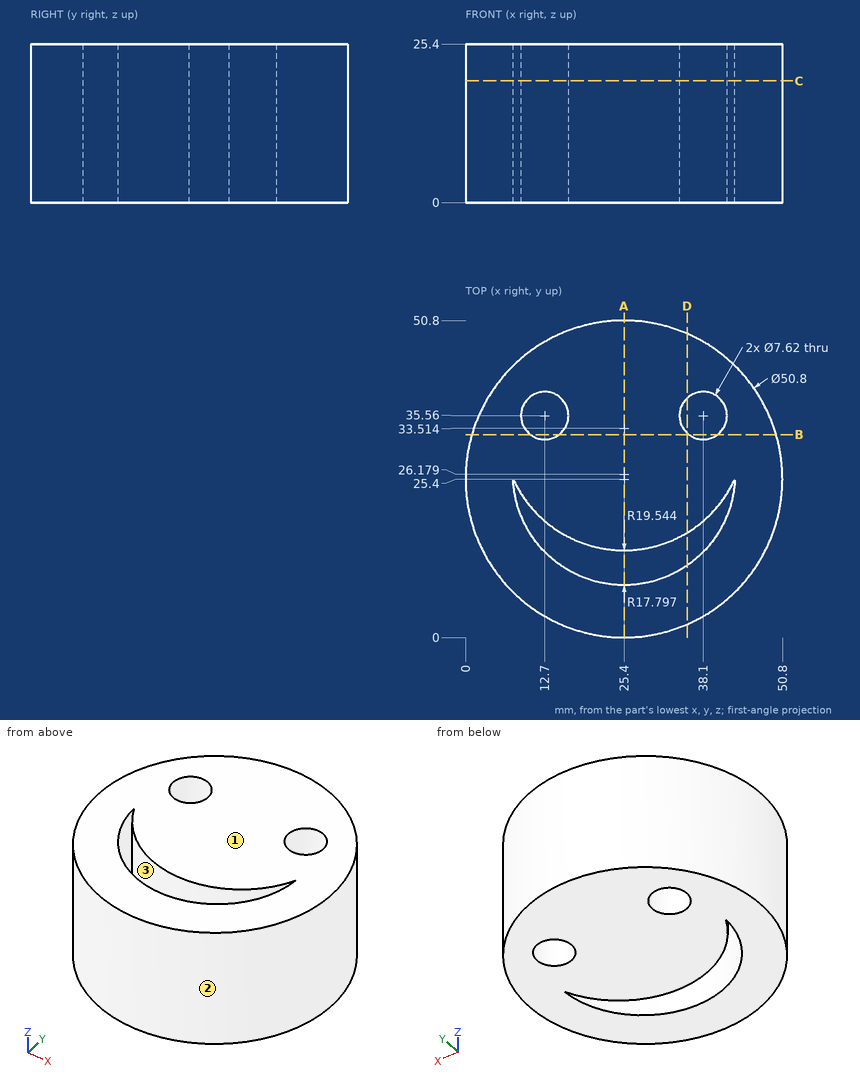
For this review, use the dimensioned drawing (mm, ordinates from the lowest corner) and the shaded views. Give positions to 0.01 mm unless a question says otherwise; leave off trailing zeros. Order: outer loops, then holes, each group sorted by start corner. A loop starts at its lowest first (then second) coordinate and runs counter-clockwise, first axis right, second up.
1) Take a section at B-B (y = 32.5). Give the boundary of the cut face in (x, z), then the cut area to 3 significant figures.
2) The part is to be moulded in two halves that separate along X. For the marked faces 1, 2 and 3, say which applies: released by +X, released by -X, zero draft, split by the parting line, or undercut.
3) Wall thickness on line 1 (Y direction, x = 12, z = 9.5) (1 decimal); line 2 (Y direction, x = 12.7, z = 13.5); line 3 (X direction, y = 16.5, z = 15.75) (1 decimal): over which ranges is each line inside the solid? List them lowest first.
4) Take a section at A-A (x = 25.4). Give the boundary of the cut face in (y, z), then the cut area to 3 significant figures.
5) Take a section at D-D (x = 35.5). Give the boundary of the cut face in (y, z) (1 decimal), then the cut area to 3 significant figures.
6) Insertion check: pin 1 (4 mm diameter, centred on y = 41, z = 19, fed in from -X); pin 2 (12 mm diameter, centred on x = 17, z = 21.5, fed in from -Y); pin 3 (6 mm diameter, centred on y = 40.5, z = 11, fed in from -X). Each pin has a flat end and moves straight along its axis. Give the tip position at first contact, or say it passes through.
7) Take a section at C-C (z = 19.5). Give the boundary of the cut face in (x, y).
Derived:
1. outline: (1.01, 0) - (10.43, 0) - (10.43, 25.4) - (1.01, 25.4) - close; (14.97, 0) - (35.83, 0) - (35.83, 25.4) - (14.97, 25.4) - close; (40.37, 0) - (49.79, 0) - (49.79, 25.4) - (40.37, 25.4) - close
1. area: 1,010 mm2
2. face 1: zero draft
2. face 2: split by the parting line
2. face 3: undercut
3. line 1: y = 3.8 to 14.5, 19.3 to 31.8, 39.3 to 47
3. line 2: y = 3.4 to 13.71, 18.66 to 31.75, 39.37 to 47.4
3. line 3: x = 1.6 to 10.5, 15.8 to 35, 40.3 to 49.2
4. outline: (0, 0) - (8.38, 0) - (8.38, 25.4) - (0, 25.4) - close; (13.97, 0) - (50.8, 0) - (50.8, 25.4) - (13.97, 25.4) - close
4. area: 1,150 mm2
5. outline: (2.1, 0) - (11.5, 0) - (11.5, 25.4) - (2.1, 25.4) - close; (16.8, 0) - (32.8, 0) - (32.8, 25.4) - (16.8, 25.4) - close; (38.3, 0) - (48.7, 0) - (48.7, 25.4) - (38.3, 25.4) - close
5. area: 909 mm2
6. pin 1: stops at x = 3.95
6. pin 2: stops at y = 0.11
6. pin 3: stops at x = 3.07
7. outline: circle Ø50.8 at (25.4, 25.4); hole (7.62, 25.4) arc R17.8 ccw to (43.18, 25.4) arc R19.54 cw to start; hole circle Ø7.62 at (12.7, 35.56); hole circle Ø7.62 at (38.1, 35.56)
